Check sheet for the modelled part. Datum: model origin and axes. Units: mm. A direction names the side the tool comes from. Give positions to 0.01 mm unless a question says otherwise; leave off trailing zeros. Write each loop counter-clockwise with the first axis right and the second up, starting at its lowest first coordinate (ties: lowest second). Pieces come first, ordered by that corner, then holes. Notation, with made-up numbers: (-38.5, 56) -> (-19.5, 56) arc R6 ccw to (-19.5, 63) -> close; hole circle Ø7 at (54, 49.5). An arc over 180 degrees is marked (long way). Return JSON: item names as keys, results as strings.
Autodesk Inventor part; units mm, degrees
ref_plane "YZ Plane" through (0, 0, 0) normal (1, 0, 0) x (0, 1, 0)
ref_plane "XZ Plane" through (0, 0, 0) normal (0, 1, 0) x (-1, 0, 0)
ref_plane "XY Plane" through (0, 0, 0) normal (0, 0, 1) x (1, 0, 0)
sketch "Sketch1" plane through (0, 0, 0) normal (0, 0, 1) x (1, 0, 0)
  circle A0 centre (0, 0) radius 15.494
  dimension "d0" = 30.988
extrude "Extrusion1" add sketch "Sketch1" along normal blind 1.27
sketch "Sketch2" plane through (0, 0, 1.27) normal (0, 0, 1) x (1, 0, 0)
  circle A0 centre (0, 0) radius 14.2875
  dimension "d3" = 28.575
extrude "Extrusion2" add sketch "Sketch2" along normal blind 6.35
sketch "Sketch3" plane through (0, 0, 7.62) normal (0, 0, 1) x (1, 0, 0)
  point P0 (0, 0)
  point P1 (0, 0)
hole "Hole1" at (0, 0, 7.62) direction (0, 0, -1) diameter 12.7 end through all
properties part number "Bearing"
(1) Cross-section at A-A on x = 0. Enter the section's corners in (y, z), then the cut area to 3 significant figures.
Reply:
{"outline": "(-15.49, 0) -> (-6.35, 0) -> (-6.35, 7.62) -> (-14.29, 7.62) -> (-14.29, 1.27) -> (-15.49, 1.27) -> close; (6.35, 0) -> (15.49, 0) -> (15.49, 1.27) -> (14.29, 1.27) -> (14.29, 7.62) -> (6.35, 7.62) -> close", "area": "124 mm^2"}
(2) Release check for a two-part mould opening along X. For faces 1 (the flat face through (6, -3, 7.62)), 2 (the cylindrical face through (6.2, 1.38, 3.76)), 3 (the cylindrical face through (-14.274, -0.628, 4.401)) record: pulls with the +X half, pulls with the -X half, needs draft (parallel to the pull), parting line crosses it, or undercut.
Reply:
{"face 1": "needs draft", "face 2": "undercut", "face 3": "parting line crosses it"}
(3) Thickness scan on L1, parallel to Y at x = 0, z = 4.75; L2, parallel to Y at x = -3, z = 4.75; L3, parallel to X at y = -4, z = 7.25. Record the ranges inside material, lowest first.
Reply:
{"L1": "-14.29 to -6.35, 6.35 to 14.29", "L2": "-13.97 to -5.6, 5.6 to 13.97", "L3": "-13.72 to -4.93, 4.93 to 13.72"}
(4) Depth check by flat-ended pin: pin 1 Ø1.5 at (y, z) = (3.5, 7) entering from +X; pin 2 Ø3 at (y, z) = (0.5, 4.5) entering from -X. Enter the tip coordinate at first touch or a pass-through.
Reply:
{"pin 1": "x = 14.02", "pin 2": "x = -14.29"}
(5) Cross-section at D-D on y = -10. Enter the section's corners in (x, z).
Reply:
{"outline": "(-11.83, 0) -> (11.83, 0) -> (11.83, 1.27) -> (10.2, 1.27) -> (10.2, 7.62) -> (-10.2, 7.62) -> (-10.2, 1.27) -> (-11.83, 1.27) -> close"}
(6) Set-up check for faces 4 (the flat face through (14, -5, 1.27)), 5 (the cylindrical face through (8.329, -13.065, 0.626)): record each of +Z, -Z, +X, -X, +Y, -Y from which the full face is reachable in a straight line by a thin tool's end or side.
Reply:
{"face 4": "+Z", "face 5": "+Z, -Z"}
